Geometry check sheet. Reference: the model listing, model coordinates, mm. Coordinates: 2 decimals unless noted, no trailing zeros. Write each loop counter-clockwise with the first axis right and the second up, starting at its lowest first coordinate (ties: lowest second). Pieces come first, ordered by that corner, then holes. Notation, with made-up numbers: M 70,-37.5 L 121,-37.5 A19 cw 121,-16.5 Z; hole C 13.5,27 d5. An arc over 180 degrees is marked long. Write each question's results on one line, items separated by ' | '.
```python
from build123d import *

# Parameters (mm, degrees)
SKETCH3_R               = 3.175
BOSS_EXTRUDE1_DEPTH     = 304.8
CHAMFER1_SIZE           = 0.635
CUT_EXTRUDE1_START      = -105.627050112
SKETCH4_R               = 3.175
CUT_EXTRUDE1_DEPTH      = 504.972949888
SKETCH5_R               = 0.5953125
CUT_EXTRUDE2_DEPTH      = 4.175
CUT_EXTRUDE2_DEPTH_BACK = 4.175


with BuildPart() as part:
    # Sketch3 → Boss-Extrude1 (new body, symmetric)
    with BuildSketch(Plane.XY):
        Circle(SKETCH3_R)
    extrude(amount=BOSS_EXTRUDE1_DEPTH, both=True)

    # Chamfer1
    chamfer1_edges = [part.edges().sort_by_distance(p)[0] for p in [
        (-3.175, 0, -304.8),
        (-3.175, 0, 304.8),
    ]]
    chamfer(chamfer1_edges, length=CHAMFER1_SIZE)

    # Sketch4 → Cut-Extrude1 (cut, through all)
    with BuildSketch(Plane.XY.offset(304.8).offset(CUT_EXTRUDE1_START)):
        Circle(SKETCH4_R)
    extrude(amount=-CUT_EXTRUDE1_DEPTH, mode=Mode.SUBTRACT)

    # Sketch5 → Cut-Extrude2 (cut, two sides)
    with BuildSketch(Plane(origin=(0, 0, 0), x_dir=(1, 0, 0), z_dir=(0, 1, 0))) as cut_extrude2_sk:
        with Locations((0, -200.760449888)):
            Circle(SKETCH5_R)
        with Locations((0, -303.2125)):
            Circle(SKETCH5_R)
    extrude(amount=CUT_EXTRUDE2_DEPTH, mode=Mode.SUBTRACT)
    extrude(cut_extrude2_sk.sketch, amount=-CUT_EXTRUDE2_DEPTH_BACK, mode=Mode.SUBTRACT)


solid = part.part
```
Q1. Sectioned sample at A-A on z = 227. Record the cut outline in (x, y) (3 decimals), and give its area (3 significant figures).
Geometry check:
outline: C 0,0 d6.35 | area: 31.7 mm2
Q2. Scan lines: probe 1 along Z at (x, y) = (0, 2.55); probe 2 along Z at (x, y) = (0.25, -1.5); probe 3 along Y at (x, z) = (1.75, 253). Record each from-to range of solid material in increasing order.
Geometry check:
probe 1: z = 199.17 to 200.17, 201.36 to 302.62, 303.81 to 304.79 | probe 2: z = 199.17 to 200.22, 201.3 to 302.67, 303.75 to 304.8 | probe 3: y = -2.65 to 2.65
Q3. Sectioned sample at B-B on y = 1.5. Give the number of separate pieces and of enclosed holes in the cut face, and give its area (3 significant figures).
Geometry check:
separate pieces: 1 | enclosed holes: 2 | area: 588 mm2
Q4. Depth check by flat-ended pin: P1, Ø1, axis at y = -1, z = 219, coming from the +X side; P2, Ø2, axis at y = -2, z = 257.5, coming from the -X side; P3, Ø1.1, axis at x = 0, z = 303.21, coming from the +Y side. Enter the tip coordinate at first touch or a pass-through.
Geometry check:
P1: stops at x = 3.14 | P2: stops at x = -3.01 | P3: passes through
